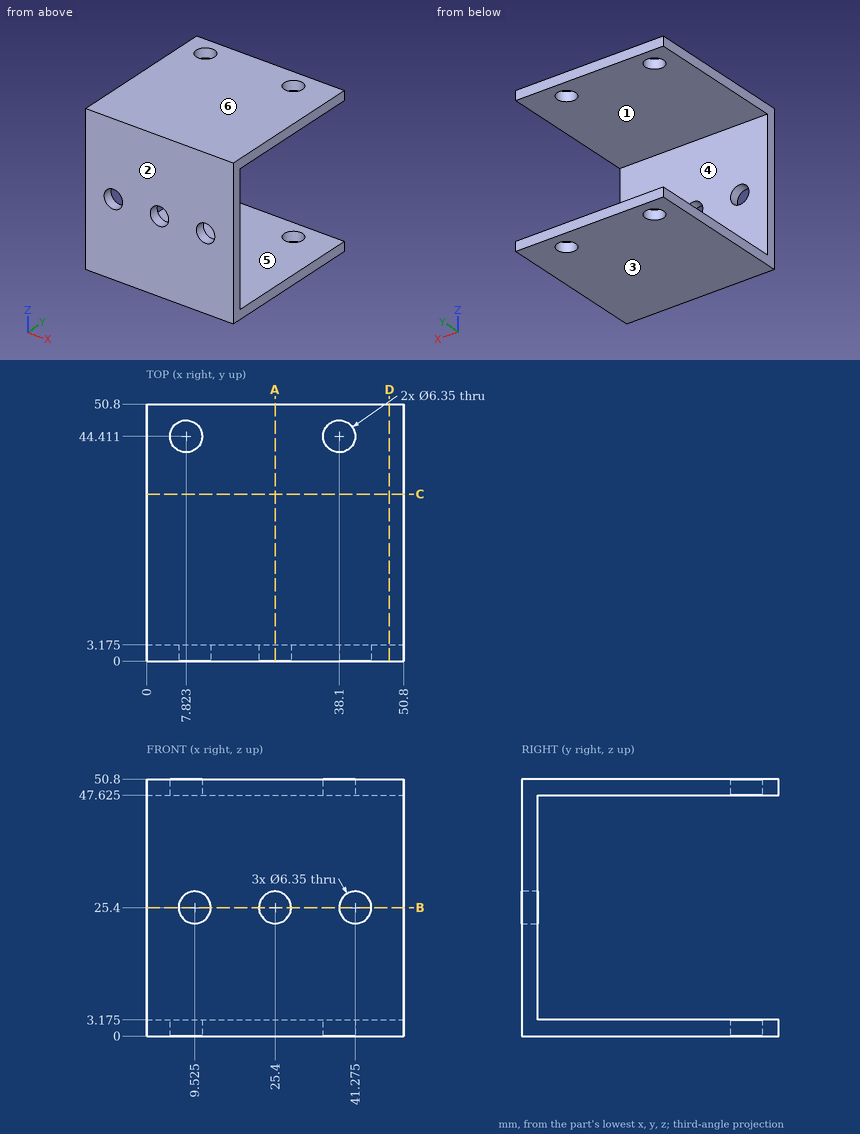
Can you work these out from the drawing? Everything is in mm from the part's minimum corner. A direction names the side the tool comes from. Round coordinates to 2 decimals unless told otherwise and drop trailing zeros. Order: outer loops, then holes, each group sorted by start corner. A loop starts at its lowest first (then second) coordinate and runs counter-clockwise, first axis right, second up. Notation, with made-up numbers: (88.5, 52) - (130.5, 52) arc R27 cw to (130.5, 85) - close; hole circle Ø9 at (39, 53.5). An arc over 180 degrees is marked (long way). Answer in a Markdown table with one row per item.
(1) If we mould it in two halves opening along Z, with no side actions, what happens to the marked faces 1, 2, 3 and 4? For each: released by +Z, released by -Z, zero draft, split by the parting line, or undercut.
From the geometry:
| item | result |
|---|---|
| face 1 | undercut |
| face 2 | zero draft |
| face 3 | released by -Z |
| face 4 | undercut |
(2) Suppose I cut it at D-D, the plane x = 48. Please give me the cut outline in (y, z) (1 decimal).
From the geometry:
| item | result |
|---|---|
| outline | (0, 0) - (50.8, 0) - (50.8, 3.2) - (3.2, 3.2) - (3.2, 47.6) - (50.8, 47.6) - (50.8, 50.8) - (0, 50.8) - close |
(3) Suppose I cut it at C-C, the plane y = 33. Please give me the cut outline in (x, z) (1 decimal).
From the geometry:
| item | result |
|---|---|
| outline | (0, 0) - (50.8, 0) - (50.8, 3.2) - (0, 3.2) - close; (0, 47.6) - (50.8, 47.6) - (50.8, 50.8) - (0, 50.8) - close |
(4) Which directions (+Z, -Z, +X, -X, +Y, -Y) give clear straight access to the entire face, cutting with the end or side of a thin tool? Please do the marked faces 5 and 6.
From the geometry:
| item | result |
|---|---|
| face 5 | +X, -X, +Y |
| face 6 | +Z, +X, -X, +Y, -Y |
(5) Please list where these lines run through material, in increasing order: L1, parallel to Y at x = 38, z = 1; L2, parallel to Z at x = 5.5, y = 28 (1 decimal); L3, parallel to Y at x = 39.5, z = 4 (1 decimal). Write a range as from..to.
From the geometry:
| item | result |
|---|---|
| L1 | y = 0..41.24, 47.58..50.8 |
| L2 | z = 0..3.2, 47.6..50.8 |
| L3 | y = 0..3.2 |
(6) Suppose I cut it at B-B, the plane z = 25.4. Count the separate pieces of the cut face and the enclosed holes in it, plus the area to 3 significant figures.
From the geometry:
| item | result |
|---|---|
| separate pieces | 4 |
| enclosed holes | 0 |
| area | 101 mm2 |
(7) For P1, Ø7.5, axis at x = 41.275, z = 25.4, coming from the +Y side (3 decimals), with a flat end and sliding along its axis, tell me the tip position at first contact or that it passes through.
From the geometry:
| item | result |
|---|---|
| P1 | stops at y = 3.175 |
(8) Suppose I cut it at A-A, the plane x = 25.4. Please give me the cut outline in (y, z) (1 decimal).
From the geometry:
| item | result |
|---|---|
| outline | (0, 0) - (50.8, 0) - (50.8, 3.2) - (3.2, 3.2) - (3.2, 22.2) - (0, 22.2) - close; (0, 28.6) - (3.2, 28.6) - (3.2, 47.6) - (50.8, 47.6) - (50.8, 50.8) - (0, 50.8) - close |
